Could you check a few things on this drawing? It's one solid part, dimensions in mm from its lowest x, y, z. A direction names the side the tool comes from. Coordinates: 2 decimals unless noted, no trailing zeros. Write each loop counter-clockwise with the first axis right and the second up, starting at its lowest first coordinate (ties: lowest second). Pieces come first, ordered by that corner, then holes.
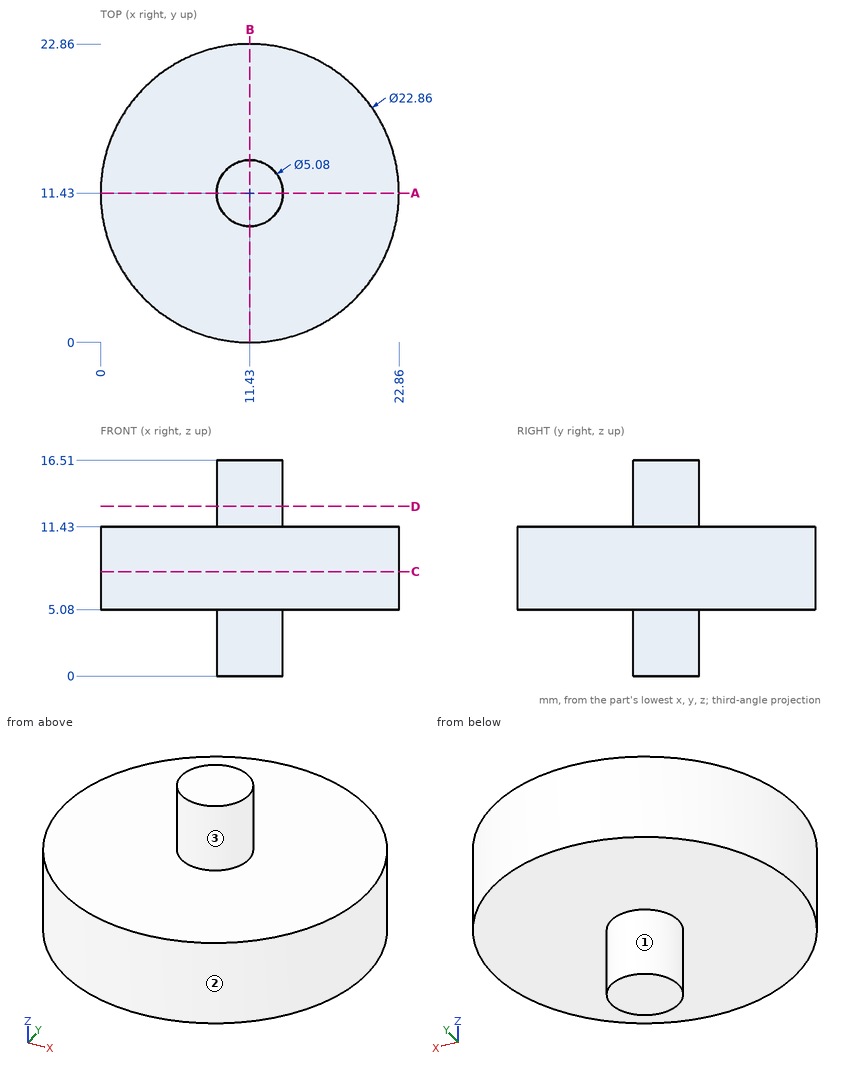
1) Will these pins go through, and if not, where does the flat tip stop? pin 1 (6 mm diameter, centred on y = 7.5, z = 6, fed in from +X); pin 2 (3 mm diameter, centred on y = 8, z = 11, fed in from -X); pin 3 (5 mm diameter, centred on y = 20, z = 5, fed in from -X).
Values follow:
pin 1: stops at x = 22.82
pin 2: stops at x = 0.16
pin 3: stops at x = 1.75
2) On a 3-axis mill with a long thin cutter (end or side, diameter ignored), from which of +Z, -Z, +X, -X, +Y, -Y can I reach the whole of each face in a straight line? I mean the marked faces 1, 2 and 3. Say none if no direction works.
Values follow:
face 1: -Z
face 2: +Z, -Z
face 3: +Z
3) Imagine slicing it at C-C on z = 8. Please give me the cut outline in (x, y), then the cut area to 3 significant figures.
Values follow:
outline: circle Ø22.86 at (11.43, 11.43)
area: 410 mm2
4) I need wall thicknesses on probe 1 along Z at (x, y) = (18, 8.25); probe 2 along X at (y, z) = (19.25, 6.25); probe 3 along Y at (x, z) = (13, 10). Which ranges of each line are inside material? Lowest first, please.
Values follow:
probe 1: z = 5.08 to 11.43
probe 2: x = 3.09 to 19.77
probe 3: y = 0.11 to 22.75
5) Imagine slicing it at A-A on y = 11.43. Please give me the cut outline in (x, z), then the cut area to 3 significant figures.
Values follow:
outline: (0, 5.08) - (8.89, 5.08) - (8.89, 0) - (13.97, 0) - (13.97, 5.08) - (22.86, 5.08) - (22.86, 11.43) - (13.97, 11.43) - (13.97, 16.51) - (8.89, 16.51) - (8.89, 11.43) - (0, 11.43) - close
area: 197 mm2
6) Imagine slicing it at D-D on z = 13. Please give me the cut outline in (x, y), then the cut area to 3 significant figures.
Values follow:
outline: circle Ø5.08 at (11.43, 11.43)
area: 20.3 mm2
